Can you work these out from the model? Positions are in its coordinate system, mm. Face numbers are marked on the shaded views. A direction names the side the tool comes from. Round coordinates to 2 decimals unless told otherwise and drop trailing zeros. Loops run counter-clockwise (first coordinate to the right, second up) from the corner with the lowest first, then second, coordinate; pieces in that order, holes last. Notation, with made-up numbers: M 78,52 L 120,52 A17 ccw 120,64 Z; hole C 10,38 d11. An arc over 180 degrees is marked long. Return JSON: item names as keys, results as strings.
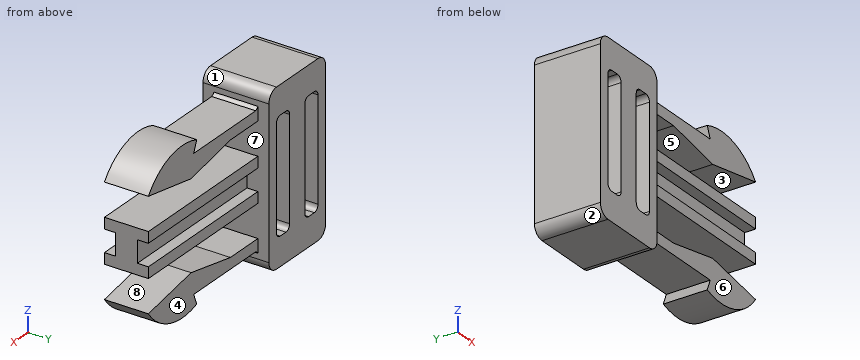
```python
from build123d import *

# Parameters (mm, degrees)
BOSS_EXTRUDE1_DEPTH = 15.24
CUT_EXTRUDE1_DEPTH  = 47.315839623
SKETCH5_W           = 36.83
SKETCH5_H           = 10.16
BOSS_EXTRUDE2_DEPTH = 10.16
SKETCH7_W           = 36.83
SKETCH7_H           = 5.08
CUT_EXTRUDE2_DEPTH  = 2.54


with BuildPart() as part:
    # Sketch1 → Boss-Extrude1 (new body)
    with BuildSketch(Plane(origin=(0, 0, 0), x_dir=(1, 0, 0), z_dir=(0, 1, 0))):
        with BuildLine():
            Line((19.05, 36.83), (19.05, 2.54))
            ThreePointArc((19.05, 2.54), (18.306051224, 0.743948776), (16.51, 0))
            Line((16.51, 0), (2.54, 0))
            ThreePointArc((2.54, 0), (0.743948776, 0.743948776), (0, 2.54))
            Line((0, 2.54), (0, 36.83))
            ThreePointArc((0, 36.83), (0.743948776, 38.626051224), (2.54, 39.37))
            Line((2.54, 39.37), (16.51, 39.37))
            ThreePointArc((16.51, 39.37), (18.306051224, 38.626051224), (19.05, 36.83))
        make_face()
    extrude(amount=BOSS_EXTRUDE1_DEPTH)

    # Sketch3 → Cut-Extrude1 (cut, through all)
    with BuildSketch(Plane(origin=(0, 15.24, 0), x_dir=(1, 0, 0), z_dir=(0, 1, 0))):
        with BuildLine():
            Line((6.985, 31.496), (6.985, 7.874))
            ThreePointArc((6.985, 7.874), (6.613025612, 6.975974388), (5.715, 6.604))
            Line((5.715, 6.604), (3.81, 6.604))
            ThreePointArc((3.81, 6.604), (2.911974388, 6.975974388), (2.54, 7.874))
            Line((2.54, 7.874), (2.54, 31.496))
            ThreePointArc((2.54, 31.496), (2.911974388, 32.394025612), (3.81, 32.766))
            Line((3.81, 32.766), (5.715, 32.766))
            ThreePointArc((5.715, 32.766), (6.613025612, 32.394025612), (6.985, 31.496))
        make_face()
        with BuildLine():
            Line((12.065, 31.496), (12.065, 7.874))
            ThreePointArc((12.065, 7.874), (12.436974388, 6.975974388), (13.335, 6.604))
            Line((13.335, 6.604), (15.24, 6.604))
            ThreePointArc((15.24, 6.604), (16.138025612, 6.975974388), (16.51, 7.874))
            Line((16.51, 7.874), (16.51, 31.496))
            ThreePointArc((16.51, 31.496), (16.138025612, 32.394025612), (15.24, 32.766))
            Line((15.24, 32.766), (13.335, 32.766))
            ThreePointArc((13.335, 32.766), (12.436974388, 32.394025612), (12.065, 31.496))
        make_face()
    extrude(amount=-CUT_EXTRUDE1_DEPTH, mode=Mode.SUBTRACT)

    # Sketch5 → Boss-Extrude2 (add)
    with BuildSketch(Plane(origin=(0, 2.54, 0), x_dir=(1, 0, 0), z_dir=(0, 1, 0))):
        with BuildLine():
            Line((19.795155373, 34.925), (40.64, 34.925))
            Line((40.64, 34.925), (39.624, 37.465))
            ThreePointArc((39.624, 37.465), (48.617910258, 37.695912826), (55.88, 32.385))
            Line((55.88, 32.385), (41.501589711, 29.845))
            Line((41.501589711, 29.845), (28.302846613, 32.385))
            Line((28.302846613, 32.385), (19.338620701, 32.385))
            Line((19.338620701, 32.385), (19.05, 32.385))
            Line((19.05, 32.385), (19.05, 35.56))
            ThreePointArc((19.05, 35.56), (19.381676592, 35.194503669), (19.795155373, 34.925))
        make_face()
        with Locations((37.465, 19.685)):
            Rectangle(SKETCH5_W, SKETCH5_H)
        with BuildLine():
            Line((19.795155373, 4.445), (40.64, 4.445))
            Line((40.64, 4.445), (39.624, 1.905))
            ThreePointArc((39.624, 1.905), (48.617910258, 1.674087174), (55.88, 6.985))
            Line((55.88, 6.985), (41.501589711, 9.525))
            Line((41.501589711, 9.525), (28.302846613, 6.985))
            Line((28.302846613, 6.985), (19.338620701, 6.985))
            Line((19.338620701, 6.985), (19.05, 6.985))
            Line((19.05, 6.985), (19.05, 3.81))
            ThreePointArc((19.05, 3.81), (19.381676592, 4.175496331), (19.795155373, 4.445))
        make_face()
    extrude(amount=BOSS_EXTRUDE2_DEPTH)

    # Sketch7 → Cut-Extrude2 (cut)
    with BuildSketch(Plane(origin=(0, 12.7, 0), x_dir=(1, 0, 0), z_dir=(0, 1, 0))):
        with Locations((37.465, 19.685)):
            Rectangle(SKETCH7_W, SKETCH7_H)
    cut_extrude2 = extrude(amount=-CUT_EXTRUDE2_DEPTH, mode=Mode.SUBTRACT)

    # Mirror1: Cut-Extrude2 across plane
    add(cut_extrude2.mirror(Plane.ZX.offset(7.62)), mode=Mode.SUBTRACT)


solid = part.part
```
Q1. If I drill on line 1 along Z through (x, y) = (33, 4.25) (3 decimals); line 2 along X through (y, z) = (3, -19.5) (3 decimals), over which ranges is the centre line in solid material (lowest first)?
Results:
{"line 1": "z = -34.925 to -31.481, -24.765 to -22.225, -17.145 to -14.605, -7.889 to -4.445", "line 2": "x = 0 to 2.54, 6.985 to 12.065, 16.51 to 19.05"}
Q2. Suppose I cut it at B-B, the plane x = 4.5. Please give me the cut outline in (y, z), plus the area to 3 significant figures.
Results:
{"outline": "M 0,-39.37 L 15.24,-39.37 L 15.24,-32.77 L 0,-32.77 Z; M 0,-6.6 L 15.24,-6.6 L 15.24,0 L 0,0 Z", "area": "201 mm2"}
Q3. Suppose I cut it at A-A, the plane z = -12.5. Please give me the cut outline in (x, y) (3 decimals), plus the area to 3 significant figures.
Results:
{"outline": "M 0,0 L 2.54,0 L 2.54,15.24 L 0,15.24 Z; M 6.985,0 L 12.065,0 L 12.065,15.24 L 6.985,15.24 Z; M 16.51,0 L 19.05,0 L 19.05,15.24 L 16.51,15.24 Z", "area": "155 mm2"}
Q4. Suppose I cut it at D-D, the plane x = 24.5. Please give me the cut outline in (y, z) (3 decimals), plus the area to 3 significant figures.
Results:
{"outline": "M 2.54,-34.925 L 12.7,-34.925 L 12.7,-32.385 L 2.54,-32.385 Z; M 2.54,-24.765 L 12.7,-24.765 L 12.7,-22.225 L 10.16,-22.225 L 10.16,-17.145 L 12.7,-17.145 L 12.7,-14.605 L 2.54,-14.605 L 2.54,-17.145 L 5.08,-17.145 L 5.08,-22.225 L 2.54,-22.225 Z; M 2.54,-6.985 L 12.7,-6.985 L 12.7,-4.445 L 2.54,-4.445 Z", "area": "129 mm2"}
Q5. I'm going to push flat-ended pins straight in: pin 1 Ø5 at (x, y) = (43, 9) entering from +Z; pin 2 Ø8 at (x, y) = (42, 12) entering from -Z; pin 3 Ø2 at (x, z) = (28.5, -23.5) entering from +Y. Where does each tip first touch, or does it pass through?
Results:
{"pin 1": "stops at z = -1.04", "pin 2": "stops at z = -38.33", "pin 3": "stops at y = 12.7"}
Q6. Suppose I cut it at C-C, the plane y = 13.5. Please give me the cut outline in (x, z) (3 decimals), plus the area to 3 significant figures.
Results:
{"outline": "M 0,-36.83 A2.54 ccw 2.54,-39.37 L 16.51,-39.37 A2.54 ccw 19.05,-36.83 L 19.05,-2.54 A2.54 ccw 16.51,0 L 2.54,0 A2.54 ccw 0,-2.54 Z; hole M 2.54,-31.496 A1.27 ccw 3.81,-32.766 L 5.715,-32.766 A1.27 ccw 6.985,-31.496 L 6.985,-7.874 A1.27 ccw 5.715,-6.604 L 3.81,-6.604 A1.27 ccw 2.54,-7.874 Z; hole M 12.065,-31.496 A1.27 ccw 13.335,-32.766 L 15.24,-32.766 A1.27 ccw 16.51,-31.496 L 16.51,-7.874 A1.27 ccw 15.24,-6.604 L 13.335,-6.604 A1.27 ccw 12.065,-7.874 Z", "area": "515 mm2"}
Q7. On a 3-axis mill with a long thin cutter (end or side, diameter ignored), from which of +Z, -Z, +X, -X, +Y, -Y can I reach the whole of each face in a straight line? I mean the marked faces 4, 5, 6, 7 and 8. Say none if no direction works.
Results:
{"face 4": "+Z, -Z, +X, +Y", "face 5": "+Y, -Y", "face 6": "+Z, -Z, +X, -Y", "face 7": "none", "face 8": "+X, +Y, -Y"}
Q8. Thinking about a two-plate mould opening in X: for the marked faces 1, 2 and 3, which applies, pulls with the +X half, pulls with the -X half, needs draft (parallel to the pull), parting line crosses it, or undercut?
Results:
{"face 1": "undercut", "face 2": "pulls with the -X half", "face 3": "pulls with the +X half"}
